Geometry check sheet. Reference: drawing and pictorial views, mm from the part's lowest x, y, z. A direction names the side the tool comes from. Give positions to 0.01 mm unless a question says otherwise; leave off trailing zeros. Loops run counter-clockwise (first coordinate to the right, second up) from the corner with the lowest first, then second, coordinate; pieces in that order, holes last. Notation, with made-up numbers: (-9.5, -13) - (21.5, -13) arc R5 cw to (21.5, -8) - close; hole circle Ø8 at (73, 41). An arc over 180 degrees is marked (long way). One line per question, with ' | ' between items. Start each with the question number.
1. Section check B-B, the plane x = 66. Enter the section's corners in (y, z).
2. Depth check by flat-ended pin: pin 1 Ø12 at (x, z) = (96, 58.5) entering from +Y. Enter the tip coordinate at first touch or a pass-through.
3. Section check C-C, the plane z = 27. Enter the section's corners in (x, y), then the cut area to 3 significant figures.
4. Thickness scan on line 1 along X through (y, z) = (27.5, 37); line 2 along Z through (x, y) = (9, 8); line 3 along Z through (x, y) = (72, 11). Record the ranges inside material, lowest first. Write a range as from..to.
5. Tool access check on the marked faces 1 and 2. Record the directions out of +Z, -Z, +X, -X, +Y, -Y that give a thin tool (end or side, any length) a straight path to the whole face; none if there is none.
6. Mould release check, pull along X, two halves, no side actions. Record for the marked faces 3, 4 and 5: +X half, -X half, draft (parallel to the pull), parting line (faces both ways), or undercut.
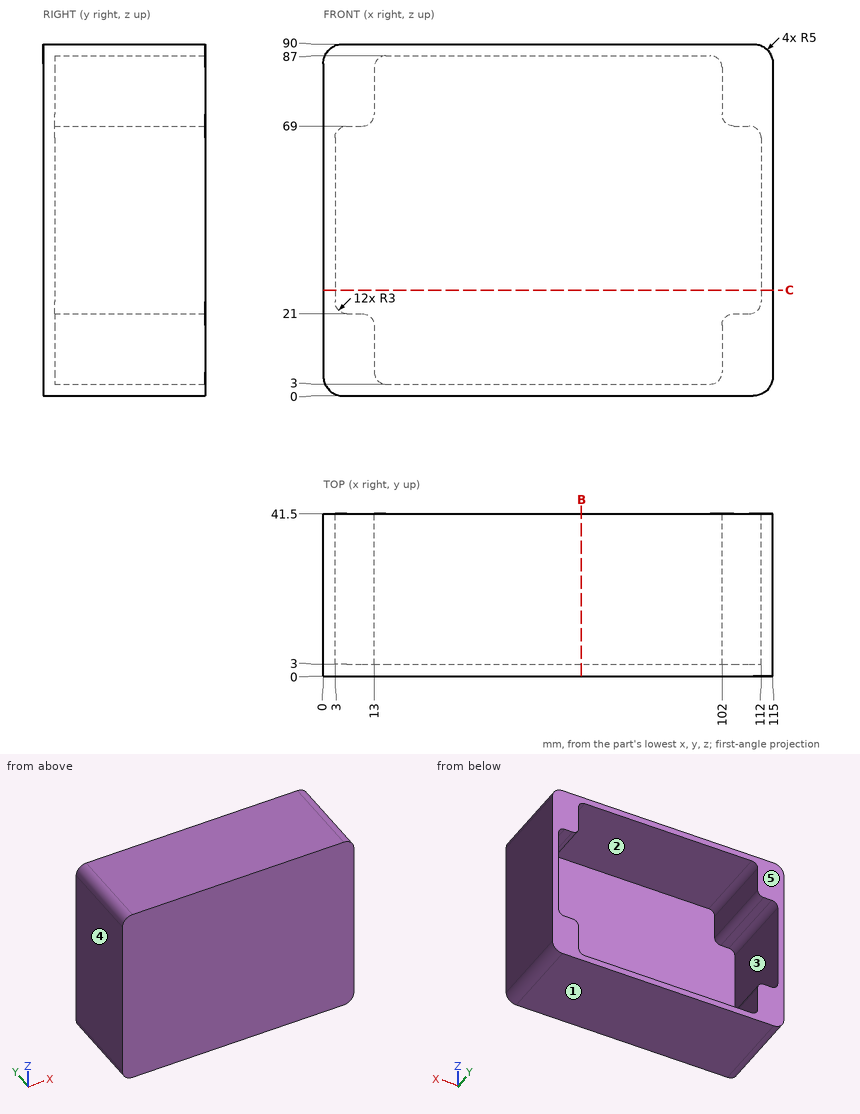
Results list:
1) outline: (0, 0) - (41.5, 0) - (41.5, 3) - (3, 3) - (3, 87) - (41.5, 87) - (41.5, 90) - (0, 90) - close
2) pin 1: y = 3
3) outline: (0, 0) - (115, 0) - (115, 41.5) - (112, 41.5) - (112, 3) - (3, 3) - (3, 41.5) - (0, 41.5) - close | area: 576 mm²
4) line 1: 0..3, 112..115 | line 2: 0..21, 69..90 | line 3: 0..3, 87..90
5) face 1: -Z, +X, -X, +Y, -Y | face 2: +Y
6) face 3: undercut | face 4: -X half | face 5: draft
